Autodesk Inventor part; units mm, degrees
ref_plane "YZ Plane" through (0, 0, 0) normal (1, 0, 0) x (0, 1, 0)
ref_plane "XZ Plane" through (0, 0, 0) normal (0, 1, 0) x (-1, 0, 0)
ref_plane "XY Plane" through (0, 0, 0) normal (0, 0, 1) x (1, 0, 0)
sketch "Sketch1" plane through (0, 0, 0) normal (0, 0, 1) x (1, 0, 0)
  circle A0 centre (0, 0) radius 9.25
  circle A1 centre (0, 30) radius 6
  circle A2 centre (20, 30) radius 6
  circle A3 centre (0, 30) radius 6.5
  circle A4 centre (20, 30) radius 6.5
  arc A5 (-1.6614, 36.2841) -> (1.6614, 36.2841) centre (0, 41) ccw
  arc A6 (-6.2729, 31.7032) -> (-4.6115, 34.5808) centre (-9.5263, 35.5) ccw
  arc A7 (-4.6115, 25.4192) -> (-6.2729, 28.2968) centre (-9.5263, 24.5) ccw
  arc A8 (1.6614, 23.7159) -> (-1.6614, 23.7159) centre (0, 19) ccw
  arc A9 (6.2729, 28.2968) -> (4.6115, 25.4192) centre (9.5263, 24.5) ccw
  arc A10 (4.6115, 34.5808) -> (6.2729, 31.7032) centre (9.5263, 35.5) ccw
  arc A11 (18.3386, 36.2841) -> (21.6614, 36.2841) centre (20, 41) ccw
  arc A12 (13.7271, 31.7032) -> (15.3885, 34.5808) centre (10.4737, 35.5) ccw
  arc A13 (15.3885, 25.4192) -> (13.7271, 28.2968) centre (10.4737, 24.5) ccw
  arc A14 (21.6614, 23.7159) -> (18.3386, 23.7159) centre (20, 19) ccw
  arc A15 (26.2729, 28.2968) -> (24.6115, 25.4192) centre (29.5263, 24.5) ccw
  arc A16 (24.6115, 34.5808) -> (26.2729, 31.7032) centre (29.5263, 35.5) ccw
  arc A17 (4.6562, 34.5353) -> (4.5, 33.9686) centre (20, 30) ccw
  arc A18 (20, 14) -> (20, 46) centre (20, 30) ccw
  line L0 (-18, 30) -> (-18, 0)
  line L1 (-2, 46) -> (20, 46)
  line L2 (-18, 0) -> (-13, 0)
  line L3 (-13, 0) -> (-13, 30)
  line L4 (-13, 30) -> (-18, 30)
  line L5 (-18, 30) -> (-18, 0)
  arc A19 (-2, 46) -> (-18, 30) centre (-2, 30) ccw
  line L6 (20, 14) -> (-13, 14)
  point P0 (15.2791, 25.532)
  point P1 (-18, 30)
  point P2 (-1.6614, 23.7159)
  point P3 (1.6614, 23.7159)
  point P4 (-6.2729, 28.2968)
  point P5 (-4.6115, 25.4192)
  point P6 (-4.6115, 34.5808)
  point P7 (4.635, 34.4629)
  point P8 (6.2729, 31.7032)
  point P9 (18.3386, 23.7159)
  point P10 (21.6614, 23.7159)
  point P11 (13.7271, 31.7032)
  point P12 (26.2729, 31.7032)
  point P13 (15.3885, 25.4192)
  point P14 (15.3885, 34.5808)
  point P15 (4.6115, 25.4192)
  dimension "d1" = 12
  dimension "d0" = 18.5
  dimension "d2" = 30
  dimension "d3" = 12
  dimension "d4" = 20
  dimension "d5" = 13
  dimension "d6" = 13
  dimension "d7" = 5
  dimension "d10" = 360
  dimension "d12" = 5
  dimension "d15" = 360
  dimension "d21" = 16
  dimension "d25" = 5
  dimension "d26" = 30
  dimension "d52" = 18
extrude "Extrusion1" add sketch "Sketch1" along normal blind 10 contours A10 A17 A3 | A9 A3 | A8 A3 | A5 A3 | A7 A3 | A6 A3 | A16 A4 | A15 A4 | A11 A4 | A14 A4 | A12 A4 | A13 A4 | L6 L3 L4 A19 L1 A18 | L3 L2 L0 L4 picked at (5.482, 33.1405)
fillet "Fillet2" radius 10 1 edges at (-13, 14, 5)
extrude "Extrusion3" add sketch "Sketch1" along normal blind 30 contours L3 L2 L0 L4
fillet "Fillet3" radius 5 3 edges at (-15.5, 30, 30) (-15.5, 0, 30) (-15.5, 0, 0)
sketch "Sketch3" plane through (-13, 4, 10) normal (1, 0, 0) x (0, 0, -1)
  line L0 (0, 26) -> (-15, 26)
  line L1 (-20, 1) -> (-20, 21)
  point P0 (10, -4)
  point P1 (-10, 16)
  dimension "d57" = 10
  dimension "d58" = 10
hole "Hole2" at (-13, 20, 20) direction (-1, 0, 0) diameter 3 end through all
sketch "Sketch4" plane through (-13, 4, 10) normal (1, 0, 0) x (0, 0, -1)
  line L0 (5, -4) -> (-15, -4)
  line L1 (-20, 1) -> (-20, 21)
  point P0 (10, -4)
  point P1 (-10, 6)
  dimension "d66" = 10
  dimension "d67" = 10
hole "Hole3" at (-13, 10, 20) direction (-1, 0, 0) diameter 3 end through all
properties part number "left_holder"
For this review, take the finished solid that the model builds, in its own axes (mm). A direction names the side the tool comes from. Give positions to 0.01 mm unless a question says otherwise; leave off trailing zeros. Write each loop counter-clockwise with the first axis right and the second up, starting at its lowest first coordinate (ties: lowest second). Pieces come first, ordered by that corner, then holes. Notation, with made-up numbers: M 73.25,29 L 99.25,29 A36 ccw 99.25,65 Z; hole C 31.25,-20.75 d4. An arc over 180 degrees is marked long. Answer as CSV lines item,"result".
1. Wall thickness on line 1 (Y direction, x = -14.3, z = 20); line 2 (Z direction, x = -14.6, y = 20); line 3 (X direction, y = 19.5, z = 24.5): over which ranges is each line inside the solid? List them lowest first.
Findings:
line 1,"y = 0 to 8.5, 11.5 to 18.5, 21.5 to 30"
line 2,"z = 0 to 18.5, 21.5 to 30"
line 3,"x = -18 to -13"
2. For pin 1 (8 mm diameter, centred on x = 12, z = 6.5, fed in from -Y); pin 2 (10 mm diameter, centred on y = 37, z = 12.5, fed in from -X); pin 3 (3 mm diameter, centred on x = -7.5, z = 5, fed in from -Y), all flat-tipped, find the tip position at first contact; note any pin that passes through.
Findings:
pin 1,"stops at y = 14"
pin 2,"stops at x = -17.78"
pin 3,"stops at y = 12"
3. Draft analysis for pull direction X (two halves, no side actions). For faces 1 (the flat face through (-18, 15, 15)), 2 (the flat face through (-16, 0, 15)), 3 (the cylindrical face through (5.238, 32.928, 4.93)), state which applies: +X half, -X half, draft (parallel to the pull), parting line (faces both ways), or undercut.
Findings:
face 1,"-X half"
face 2,"draft"
face 3,"undercut"
4. Consider section C-C, the plane x = 3. Write out the cut boundary in (y, z), then the cut area to 3 significant figures.
Findings:
outline,"M 14,0 L 24.23,0 L 24.23,10 L 14,10 Z; M 35.77,0 L 46,0 L 46,10 L 35.77,10 Z"
area,"205 mm2"
5. For faces 4 (the flat face through (-15, 30, 17)), 5 (the cylindrical face through (23.3, 24.4, 4.9)), 6 (the cylindrical face through (36, 30, 5)), 7 (the flat face through (9, 14, 5)), list the 3-axis set-ups (+Z, -Z, +X, -X, +Y, -Y) from which the entire face can be reached by the end or side of a thin tool; tool diameter is ignored.
Findings:
face 4,"+Z, +X, -X, +Y"
face 5,"+Z, -Z"
face 6,"+Z, -Z, +X"
face 7,"+Z, -Z, +X, -Y"
6. Consider section A-A, the plane y = 20. Write out the cut boundary in (x, z).
Findings:
outline,"M -18,0 L 32.49,0 L 32.49,10 L -13,10 L -13,18.5 L -18,18.5 Z; M -18,21.5 L -13,21.5 L -13,30 L -18,30 Z"
7. Consider section D-D, the plane y = 10. Write out the cut boundary in (x, z), then the cut area to 3 significant figures.
Findings:
outline,"M -18,0 L -11,0 L -11,10 L -13,10 L -13,18.5 L -18,18.5 Z; M -18,21.5 L -13,21.5 L -13,30 L -18,30 Z"
area,"155 mm2"
8. Consider section B-B, the plane z = 20. Write out the cut boundary in (x, y), then the cut area to 3 significant figures.
Findings:
outline,"M -18,0 L -13,0 L -13,8.5 L -18,8.5 Z; M -18,11.5 L -13,11.5 L -13,18.5 L -18,18.5 Z; M -18,21.5 L -13,21.5 L -13,30 L -18,30 Z"
area,"120 mm2"
